Source: CAD feature listing. Evaluate the final solid. Frame: model axes, mm. A direction names the side the tool comes from. Give positions to 0.01 mm unless a question says otherwise; leave off trailing zeros. Order: outer loops, then holes, each group sorted by start corner. A loop starts at its lowest first (then second) coordinate and runs counter-clockwise, first axis right, second up.
```python
from build123d import *

# Parameters (mm, degrees)
ESQUISSE1_W                = 20
ESQUISSE1_H                = 70
BOSS_EXTRU_1_DEPTH         = 6
ESQUISSE2_W                = 8
ESQUISSE2_H                = 9
ESQUISSE2_W_2              = 7
ENL_V_MAT_EXTRU_1_DEPTH    = 3
ESQUISSE3_W                = 7
ESQUISSE3_H                = 6
BOSS_EXTRU_2_DEPTH         = 6
ESQUISSE4_R                = 2.5
ENL_V_MAT_EXTRU_2_DEPTH    = 10
R_P_TITION_LIN_AIRE1_COUNT = 2
R_P_TITION_LIN_AIRE1_PITCH = 9


with BuildPart() as part:
    # Esquisse1 → Boss.-Extru.1 (new body)
    with BuildSketch(Plane.XY):
        with Locations((10, 35)):
            Rectangle(ESQUISSE1_W, ESQUISSE1_H)
    extrude(amount=BOSS_EXTRU_1_DEPTH)

    # Esquisse2 → Enlèv. mat.-Extru.1 (cut)
    with BuildSketch(Plane(origin=(0, 0, 0), x_dir=(-1, 0, 0), z_dir=(0, 0, -1))):
        with Locations((-4, 30)):
            Rectangle(ESQUISSE2_W, ESQUISSE2_H)
        with Locations((-16.5, 30)):
            Rectangle(ESQUISSE2_W_2, ESQUISSE2_H)
    extrude(amount=-ENL_V_MAT_EXTRU_1_DEPTH, mode=Mode.SUBTRACT)

    # Esquisse3 → Boss.-Extru.2 (add)
    with BuildSketch(Plane.XZ):
        with Locations((8.5, 3)):
            Rectangle(ESQUISSE3_W, ESQUISSE3_H)
    extrude(amount=BOSS_EXTRU_2_DEPTH)

    # Esquisse4 → Enlèv. mat.-Extru.2 (cut)
    with BuildSketch(Plane(origin=(0, 70, 0), x_dir=(1, 0, 0), z_dir=(0, 1, 0))):
        with Locations(Location((5, -3, 0), (0, 0, 270))):
            Circle(ESQUISSE4_R)
    enl_v_mat_extru_2 = extrude(amount=-ENL_V_MAT_EXTRU_2_DEPTH, mode=Mode.SUBTRACT)

    # Répétition linéaire1: Enlèv. mat.-Extru.2 ×2
    with Locations(*[(i * R_P_TITION_LIN_AIRE1_PITCH, 0, 0) for i in range(1, R_P_TITION_LIN_AIRE1_COUNT)]):
        add(enl_v_mat_extru_2, mode=Mode.SUBTRACT)


solid = part.part
```
1) Reachability of faces 1 (the flat face through (2, 0, 3)), 2 (the flat face through (12, -3, 3)), 3 (the flat face through (13, 30, 1)) from +Z, -Z, +X, -X, +Y, -Y: full face, straight path, thin tool, end or side. Return the list, or none.
Report:
face 1: +Z, -Z, -X, -Y
face 2: +Z, -Z, +X, -Y
face 3: -Z, +X
2) Draft query along X for faces 4 (the flat face through (14, 60, 3)), 5 (the flat face through (0, 35, 3)), 6 (the flat face through (5, 60, 3)), 7 (the flat face through (10, 33, 0)). Return one class per face: +X half, -X half, draft (parallel to the pull), parting line (faces both ways), or undercut.
Report:
face 4: undercut
face 5: -X half
face 6: undercut
face 7: draft
3) Section query C-C, the plane z = 1.8. Return the cut outline in (x, y).
Report:
outline: (0, 0) - (5, 0) - (5, -6) - (12, -6) - (12, 0) - (20, 0) - (20, 25.5) - (13, 25.5) - (13, 34.5) - (20, 34.5) - (20, 70) - (16.19, 70) - (16.19, 60) - (11.81, 60) - (11.81, 70) - (7.19, 70) - (7.19, 60) - (2.81, 60) - (2.81, 70) - (0, 70) - (0, 34.5) - (8, 34.5) - (8, 25.5) - (0, 25.5) - close
4) Material intervals for L1, parallel to X at y = 64, z = 3; L2, parallel to Y at x = 7.25, z = 2.35; L3, parallel to X at y = 34, z = 1.55, sorted ascending.
Report:
L1: x = 0 to 2.5, 7.5 to 11.5, 16.5 to 20
L2: y = -6 to 25.5, 34.5 to 60
L3: x = 8 to 13
5) Section query D-D, the plane y = 31. Return the cut outline in (x, z), and give its area (3 significant figures).
Report:
outline: (0, 3) - (8, 3) - (8, 0) - (13, 0) - (13, 3) - (20, 3) - (20, 6) - (0, 6) - close
area: 75.0 mm2
6) Section query B-B, the plane x = 14. Return the cut outline in (y, z), and give its area (3 significant figures).
Report:
outline: (0, 0) - (25.5, 0) - (25.5, 3) - (34.5, 3) - (34.5, 0) - (70, 0) - (70, 0.5) - (60, 0.5) - (60, 5.5) - (70, 5.5) - (70, 6) - (0, 6) - close
area: 343 mm2
7) Pin query (flat end, axial travel): pin 1 (1.5 mm diameter, centred on x = 2.5, z = 3, fed in from -Y); pin 2 (1.5 mm diameter, centred on y = 43.5, z = 2.5, fed in from -X); pin 3 (0.9 mm diameter, centred on x = 15, z = 2, fed in from +Y); pin 4 (3 mm diameter, centred on y = -2, z = 2, fed in from +X). Return the tip coordinate at first contact, or that it passes through.
Report:
pin 1: stops at y = 0
pin 2: stops at x = 0
pin 3: stops at y = 60
pin 4: stops at x = 12
8) Section query A-A, the plane y = 61. Return the cut outline in (x, z), and give its area (3 significant figures).
Report:
outline: (0, 0) - (20, 0) - (20, 6) - (0, 6) - close; hole circle Ø5 at (5, 3); hole circle Ø5 at (14, 3)
area: 80.7 mm2
